from build123d import *

# Parameters (mm, degrees)
EXTRUDE_1_DEPTH     = 32
SKETCH_2_W          = 12
SKETCH_2_H          = 3.140299871
SKETCH_2_W_2        = 15
SKETCH_2_H_2        = 5
EXTRUDE_2_DEPTH     = 32
SKETCH_3_W          = 12
SKETCH_3_H          = 9
EXTRUDE_3_DEPTH     = 19
CUT_EXTRUDE_1_DEPTH = 15
FILLET_1_R          = 2
CUT_EXTRUDE_2_REACH = 104.689
SKETCH_5_R          = 1.711419382


with BuildPart() as part:
    # ｽｹｯﾁ1 → ﾎﾞｽ - 押し出し1 (new body)
    with BuildSketch(Plane.XY):
        with BuildLine():
            Line((-57.15, 0), (-62.15, 0))
            ThreePointArc((-62.15, 0), (0, 62.15), (62.15, 0))
            Line((62.15, 0), (57.15, 0))
            ThreePointArc((57.15, 0), (0, 57.15), (-57.15, 0))
        make_face()
    extrude(amount=EXTRUDE_1_DEPTH)

    # ｽｹｯﾁ2 → ﾎﾞｽ - 押し出し2 (add)
    with BuildSketch(Plane.XY.offset(32)):
        with Locations((0, 63.429850065)):
            Rectangle(SKETCH_2_W, SKETCH_2_H)
        with Locations((69.448547198, 2.5)):
            Rectangle(SKETCH_2_W_2, SKETCH_2_H_2)
        with Locations((-69.448547198, 2.5)):
            Rectangle(SKETCH_2_W_2, SKETCH_2_H_2)
    extrude(amount=-EXTRUDE_2_DEPTH)

    # ｽｹｯﾁ3 → ﾎﾞｽ - 押し出し3 (add)
    with BuildSketch(Plane.ZY.offset(76.948547198)):
        with Locations((16, 4.5)):
            Rectangle(SKETCH_3_W, SKETCH_3_H)
    extrude(amount=-EXTRUDE_3_DEPTH)

    # ｽｹｯﾁ4 → ｶｯﾄ - 押し出し1 (cut)
    with BuildSketch(Plane.ZY.offset(76.948547198)):
        with BuildLine():
            Line((10, 0), (22, 0))
            ThreePointArc((22, 0), (16, 6), (10, 0))
        make_face()
    extrude(amount=-CUT_EXTRUDE_1_DEPTH, mode=Mode.SUBTRACT)

    # ﾌｨﾚｯﾄ1
    fillet_1_edges = [part.edges().sort_by_distance(p)[0] for p in [
        (-69.22172268, 9, 10),
        (-69.22172268, 9, 22),
    ]]
    fillet(fillet_1_edges, radius=FILLET_1_R)

    # ｽｹｯﾁ5 → ｶｯﾄ - 押し出し2 (cut, up to next)
    with BuildSketch(Plane(origin=(0, 5, 0), x_dir=(1, 0, 0), z_dir=(0, 1, 0)), mode=Mode.PRIVATE) as cut_extrude_2_sk1:
        with Locations(Location((-69.448547198, -5, 0), (0, 0, 180))):
            Circle(SKETCH_5_R)
    cut_extrude_2_tool1 = extrude(cut_extrude_2_sk1.sketch, amount=-CUT_EXTRUDE_2_REACH, mode=Mode.PRIVATE) & part.part
    # ｽｹｯﾁ5 → ｶｯﾄ - 押し出し2 (cut, up to next)
    with BuildSketch(Plane(origin=(0, 5, 0), x_dir=(1, 0, 0), z_dir=(0, 1, 0)), mode=Mode.PRIVATE) as cut_extrude_2_sk2:
        with Locations(Location((-69.448547198, -27, 0), (0, 0, 180))):
            Circle(SKETCH_5_R)
    cut_extrude_2_tool2 = extrude(cut_extrude_2_sk2.sketch, amount=-CUT_EXTRUDE_2_REACH, mode=Mode.PRIVATE) & part.part
    # ｽｹｯﾁ5 → ｶｯﾄ - 押し出し2 (cut, up to next)
    with BuildSketch(Plane(origin=(0, 5, 0), x_dir=(1, 0, 0), z_dir=(0, 1, 0)), mode=Mode.PRIVATE) as cut_extrude_2_sk3:
        with Locations(Location((69.448547198, -27, 0), (0, 0, 180))):
            Circle(SKETCH_5_R)
    cut_extrude_2_tool3 = extrude(cut_extrude_2_sk3.sketch, amount=-CUT_EXTRUDE_2_REACH, mode=Mode.PRIVATE) & part.part
    # ｽｹｯﾁ5 → ｶｯﾄ - 押し出し2 (cut, up to next)
    with BuildSketch(Plane(origin=(0, 5, 0), x_dir=(1, 0, 0), z_dir=(0, 1, 0)), mode=Mode.PRIVATE) as cut_extrude_2_sk4:
        with Locations(Location((69.448547198, -5, 0), (0, 0, 180))):
            Circle(SKETCH_5_R)
    cut_extrude_2_tool4 = extrude(cut_extrude_2_sk4.sketch, amount=-CUT_EXTRUDE_2_REACH, mode=Mode.PRIVATE) & part.part
    add(cut_extrude_2_tool1.solids().sort_by_distance((-69.448547, 5, 5))[0], mode=Mode.SUBTRACT)
    add(cut_extrude_2_tool2.solids().sort_by_distance((-69.448547, 5, 27))[0], mode=Mode.SUBTRACT)
    add(cut_extrude_2_tool3.solids().sort_by_distance((69.448547, 5, 27))[0], mode=Mode.SUBTRACT)
    add(cut_extrude_2_tool4.solids().sort_by_distance((69.448547, 5, 5))[0], mode=Mode.SUBTRACT)


solid = part.part
CAD build for the part. Positions are in the model's coordinates, mm. A direction names the side the tool comes from. Coordinates: 2 decimals unless noted, no trailing zeros. Write each loop counter-clockwise with the first axis right and the second up, starting at its lowest first coordinate (ties: lowest second). Pieces come first, ordered by that corner, then holes. Notation, with made-up numbers: (44, 73.25) - (79, 73.25) arc R13 cw to (79, 85.25) - close; hole circle Ø2 at (1.5, 55). An arc over 180 degrees is marked (long way). Use a Markdown table: item, result. Add a question column.
Item 1: Band-saw the part on B-B, the plane y = 20. Give the cut face in (x, z).
Item 2: 3-axis set-ups, long thin cutter, end or side, ignore diameter. For faces 5 (the face through (0, 65, 16)), 6 (the face through (-71.2, 5, 4)), 7 (the face through (-71.2, 5, 28.2)), 8 (the face through (69, 5, 16)), 9 (the face through (-61.949, 2, 16)): which of +Z, -Z, +X, -X, +Y, -Y reach the whole face in a straight line?
Item 3: Flat gauge pins, fed straight in: pin 1 (3 mm diameter, centred on y = 54, z = 14, fed in from -X); pin 2 (5 mm diameter, centred on y = 2.5, z = 14.5, fed in from -X); pin 3 (4 mm diameter, centred on x = 28.5, z = 8.5, fed in from -Y); pin 4 (2 mm diameter, centred on x = 69.45, z = 5, fed in from -Y). Where does each tip first touch, or does it go through?
Item 4: Band-saw the part on D-D, the plane y = 43.5. Give the cut face in (x, z).
Item 5: Band-saw the part on A-A, the plane z = 27. Give the cut face in (x, y).
Item 6: Mould opens along X. For faces 1 (the face through (67.87, 2.54, 26.34)), 2 (the face through (-69, 9, 16)), 3 (the face through (-67.74, 2.54, 5.08)), 4 (the face through (43.873, 44.02, 15.776)) say: pulls with the +X half, pulls with the -X half, needs draft (parallel to the pull), parting line crosses it, or undercut.
Item 7: Band-saw the part on C-C, the plane z = 16. Give the cut face in (x, y).
Item 8: Drill centre lines: L1, parallel to X at y = 3, z = 4.5; L2, parallel to X at y = 13, z = 3; L3, parallel to X at y = 39.5, z = 7. Where is each one in solid material? Low to high. Write a range as from..to.
Numbers:
| question | item | result |
|---|---|---|
| 1 | outline | (-58.84, 0) - (-53.54, 0) - (-53.54, 32) - (-58.84, 32) - close; (53.54, 0) - (58.84, 0) - (58.84, 32) - (53.54, 32) - close |
| 2 | face 5 | +Z, -Z, +X, -X, +Y |
| 2 | face 6 | -Z, -X, +Y |
| 2 | face 7 | +Z, -X, +Y |
| 2 | face 8 | +Z, -Z, +X, +Y |
| 2 | face 9 | -X, -Y |
| 3 | pin 1 | x = -33.26 |
| 3 | pin 2 | x = -61.95 |
| 3 | pin 3 | y = 48.33 |
| 3 | pin 4 | through |
| 4 | outline | (-44.39, 0) - (-37.07, 0) - (-37.07, 32) - (-44.39, 32) - close; (37.07, 0) - (44.39, 0) - (44.39, 32) - (37.07, 32) - close |
| 5 | outline | (-76.95, 0) - (-71.16, 0) - (-71.16, 5) - (-76.95, 5) - close; (-67.74, 0) - (-57.15, 0) arc R57.15 cw to (57.15, 0) - (67.74, 0) - (67.74, 5) - (61.95, 5) arc R62.15 ccw to (6, 61.86) - (6, 65) - (-6, 65) - (-6, 61.86) arc R62.15 ccw to (-61.95, 5) - (-67.74, 5) - close; (71.16, 0) - (76.95, 0) - (76.95, 5) - (71.16, 5) - close |
| 6 | face 1 | undercut |
| 6 | face 2 | needs draft |
| 6 | face 3 | undercut |
| 6 | face 4 | pulls with the +X half |
| 7 | outline | (-76.95, 6) - (-61.95, 6) - (-61.95, 0) - (-57.15, 0) arc R57.15 cw to (57.15, 0) - (76.95, 0) - (76.95, 5) - (61.95, 5) arc R62.15 ccw to (6, 61.86) - (6, 65) - (-6, 65) - (-6, 61.86) arc R62.15 ccw to (-61.49, 9) - (-76.95, 9) - close |
| 8 | L1 | -76.95..-71.09, -67.81..-57.07, 57.07..67.81, 71.09..76.95 |
| 8 | L2 | -60.78..-55.65, 55.65..60.78 |
| 8 | L3 | -47.98..-41.3, 41.3..47.98 |
